Autodesk Inventor part; units mm, degrees
ref_plane "YZ Plane" through (0, 0, 0) normal (1, 0, 0) x (0, 1, 0)
ref_plane "XZ Plane" through (0, 0, 0) normal (0, 1, 0) x (-1, 0, 0)
ref_plane "XY Plane" through (0, 0, 0) normal (0, 0, 1) x (1, 0, 0)
sketch "Sketch1" plane through (0, 0, 0) normal (0, 0, 1) x (1, 0, 0)
  line L0 (2, -6) -> (2, -9) construction
  line L1 (-22, -9) -> (-22, -6) construction
  line L2 (20, -40) -> (20, -3) construction
  line L3 (-40, -3) -> (-40, -40) construction
  line L4 (20, -9) -> (-40, -9)
  line L5 (-40, -9) -> (-40, -6)
  line L6 (-40, -6) -> (20, -6)
  line L7 (20, -6) -> (20, -9)
  point P0 (0, 0)
  dimension "d0" = 3
  dimension "d1" = 60
extrude "Extrusion1" add sketch "Sketch1" along normal blind 63.5
sketch "Sketch2" plane through (0, 0, 63.5) normal (0, 0, 1) x (1, 0, 0)
  line L0 (-22, -9) -> (-22, -6)
  line L1 (2, -9) -> (-22, -9)
  line L2 (-22, -6) -> (2, -6)
  line L3 (2, -6) -> (2, -9)
  point P0 (0, 0)
extrude "Extrusion2" add sketch "Sketch2" along normal blind 3
ref_plane "Work Plane1" through (0, 0, 31.75) normal (0, 0, 1) x (1, 0, 0)
mirror "Mirror1" about plane through (0, 0, 31.75) normal (0, 0, 1) of "Extrusion2"
sketch "Sketch3" plane through (20, -9, 0) normal (0, -1, 0) x (1, 0, 0)
  circle A0 centre (-7.5, 31.75) radius 1.5
  circle A1 centre (-20, 44.25) radius 1.5
  circle A2 centre (-20, 19.25) radius 1.5
  point P0 (-20, 0)
extrude "Extrusion3" cut sketch "Sketch3" against normal blind 3
properties part number "Pan base cross bar"
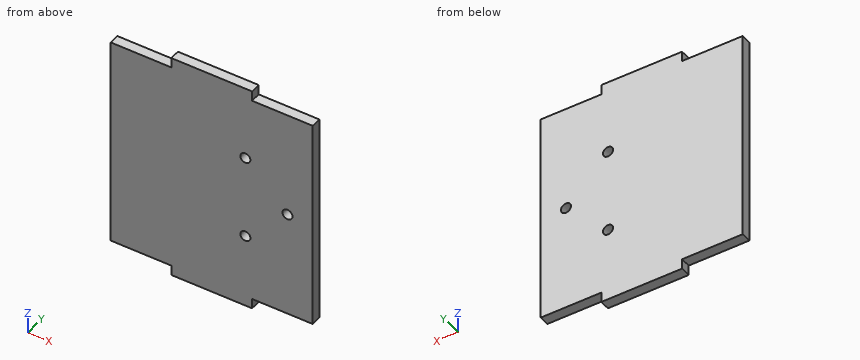
Geometry check sheet. Reference: the model listing, model coordinates, mm. Coordinates: 2 decimals unless noted, no trailing zeros. Order: outer loops, then holes, each group sorted by start corner. A loop starts at its lowest first (then second) coordinate and runs counter-clockwise, first axis right, second up. Notation, with made-up numbers: M 12,25 L 40,25 A17 cw 40,33 Z; hole C 40.5,43.25 d1. An arc over 180 degrees is marked long. Use CSV: the item, a comma, the result in double quotes.
Item 1: Thickness scan on line 1 along Z through (x, y) = (0, -7.8); line 2 along Z through (x, y) = (12.5, -7); line 3 along Z through (x, y) = (-30, -8.5). Record the ranges inside material, lowest first.
Returned:
line 1,"z = -3 to 17.75, 20.75 to 42.75, 45.75 to 66.5"
line 2,"z = 0 to 30.25, 33.25 to 63.5"
line 3,"z = 0 to 63.5"
Item 2: Cross-section at A-A on x = 0. Record the cut outline in (y, z).
Returned:
outline,"M -9,-3 L -6,-3 L -6,17.75 L -9,17.75 Z; M -9,20.75 L -6,20.75 L -6,42.75 L -9,42.75 Z; M -9,45.75 L -6,45.75 L -6,66.5 L -9,66.5 Z"
Item 3: Cross-section at C-C on x = 12.5. Record the cut outline in (y, z), then the cut area to 4 significant figures.
Returned:
outline,"M -9,0 L -6,0 L -6,30.25 L -9,30.25 Z; M -9,33.25 L -6,33.25 L -6,63.5 L -9,63.5 Z"
area,"181.5 mm2"
Item 4: Gauge pin test, flat ends, axial feed: pin 1 Ø0.9 at (x, y) = (12, -7) entering from -Z; pin 2 Ø1.5 at (y, z) = (-8, 65.5) entering from -X; pin 3 Ø1.5 at (y, z) = (-7, -2) entering from +X. Record the tip position at first contact, or that the pin passes through.
Returned:
pin 1,"stops at z = 0"
pin 2,"stops at x = -22"
pin 3,"stops at x = 2"
Item 5: Cross-section at B-B on z = 19.25. Record the cut outline in (x, y).
Returned:
outline,"M -40,-9 L -1.5,-9 L -1.5,-6 L -40,-6 Z; M 1.5,-9 L 20,-9 L 20,-6 L 1.5,-6 Z"
Item 6: Cross-section at D-D on y = -6.8. Record the cut outline in (x, z).
Returned:
outline,"M -40,0 L -22,0 L -22,-3 L 2,-3 L 2,0 L 20,0 L 20,63.5 L 2,63.5 L 2,66.5 L -22,66.5 L -22,63.5 L -40,63.5 Z; hole C 0,19.25 d3; hole C 0,44.25 d3; hole C 12.5,31.75 d3"
